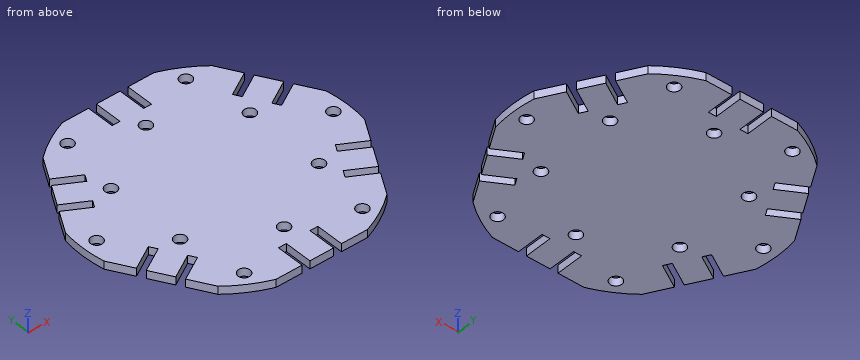
from build123d import *

# Parameters (mm, degrees)
MODEL_R             = 1.5
BOSS_EXTRUDE1_DEPTH = 2


with BuildPart() as part:
    # Model → Boss-Extrude1 (new body)
    with BuildSketch(Plane.XY):
        with BuildLine():
            Line((-18.701410202, -16.570766906), (-19.701410202, -14.838716098))
            Line((-19.701410202, -14.838716098), (-25.711054778, -18.308386013))
            Line((-25.711054778, -18.308386013), (-28.711054778, -13.11223359))
            Line((-28.711054778, -13.11223359), (-22.701410202, -9.642563676))
            Line((-22.701410202, -9.642563676), (-23.701410202, -7.910512868))
            Line((-23.701410202, -7.910512868), (-29.711054778, -11.380182782))
            Line((-29.711054778, -11.380182782), (-33.02041498, -5.648202773))
            ThreePointArc((-33.02041498, -5.648202773), (-33.5, 0), (-33.02041498, 5.648202773))
            Line((-33.02041498, 5.648202773), (-29.711054778, 11.380182782))
            Line((-29.711054778, 11.380182782), (-23.701410202, 7.910512868))
            Line((-23.701410202, 7.910512868), (-22.701410202, 9.642563676))
            Line((-22.701410202, 9.642563676), (-28.711054778, 13.11223359))
            Line((-28.711054778, 13.11223359), (-25.711054778, 18.308386013))
            Line((-25.711054778, 18.308386013), (-19.701410202, 14.838716098))
            Line((-19.701410202, 14.838716098), (-18.701410202, 16.570766906))
            Line((-18.701410202, 16.570766906), (-24.711054778, 20.04043682))
            Line((-24.711054778, 20.04043682), (-21.401694577, 25.77241683))
            ThreePointArc((-21.401694577, 25.77241683), (-16.75, 29.011851027), (-11.618720403, 31.420619602))
            Line((-11.618720403, 31.420619602), (-5, 31.420619602))
            Line((-5, 31.420619602), (-5, 24.481279774))
            Line((-5, 24.481279774), (-3, 24.481279774))
            Line((-3, 24.481279774), (-3, 31.420619602))
            Line((-3, 31.420619602), (3, 31.420619602))
            Line((3, 31.420619602), (3, 24.481279774))
            Line((3, 24.481279774), (5, 24.481279774))
            Line((5, 24.481279774), (5, 31.420619602))
            Line((5, 31.420619602), (11.618720403, 31.420619602))
            ThreePointArc((11.618720403, 31.420619602), (16.75, 29.011851027), (21.401694577, 25.77241683))
            Line((21.401694577, 25.77241683), (24.711054778, 20.04043682))
            Line((24.711054778, 20.04043682), (18.701410202, 16.570766906))
            Line((18.701410202, 16.570766906), (19.701410202, 14.838716098))
            Line((19.701410202, 14.838716098), (25.711054778, 18.308386013))
            Line((25.711054778, 18.308386013), (28.711054778, 13.11223359))
            Line((28.711054778, 13.11223359), (22.701410202, 9.642563676))
            Line((22.701410202, 9.642563676), (23.701410202, 7.910512868))
            Line((23.701410202, 7.910512868), (29.711054778, 11.380182782))
            Line((29.711054778, 11.380182782), (33.02041498, 5.648202773))
            ThreePointArc((33.02041498, 5.648202773), (33.5, 0), (33.02041498, -5.648202773))
            Line((33.02041498, -5.648202773), (29.711054778, -11.380182782))
            Line((29.711054778, -11.380182782), (23.701410202, -7.910512868))
            Line((23.701410202, -7.910512868), (22.701410202, -9.642563676))
            Line((22.701410202, -9.642563676), (28.711054778, -13.11223359))
            Line((28.711054778, -13.11223359), (25.711054778, -18.308386013))
            Line((25.711054778, -18.308386013), (19.701410202, -14.838716098))
            Line((19.701410202, -14.838716098), (18.701410202, -16.570766906))
            Line((18.701410202, -16.570766906), (24.711054778, -20.04043682))
            Line((24.711054778, -20.04043682), (21.401694577, -25.77241683))
            ThreePointArc((21.401694577, -25.77241683), (16.75, -29.011851027), (11.618720403, -31.420619602))
            Line((11.618720403, -31.420619602), (5, -31.420619602))
            Line((5, -31.420619602), (5, -24.481279774))
            Line((5, -24.481279774), (3, -24.481279774))
            Line((3, -24.481279774), (3, -31.420619602))
            Line((3, -31.420619602), (-3, -31.420619602))
            Line((-3, -31.420619602), (-3, -24.481279774))
            Line((-3, -24.481279774), (-5, -24.481279774))
            Line((-5, -24.481279774), (-5, -31.420619602))
            Line((-5, -31.420619602), (-11.618720403, -31.420619602))
            ThreePointArc((-11.618720403, -31.420619602), (-16.75, -29.011851027), (-21.401694577, -25.77241683))
            Line((-21.401694577, -25.77241683), (-24.711054778, -20.04043682))
            Line((-24.711054778, -20.04043682), (-18.701410202, -16.570766906))
        make_face()
        with Locations((-17.610482102, -10.167416582)):
            Circle(MODEL_R, mode=Mode.SUBTRACT)
        with Locations((-17.610482102, 10.167416582)):
            Circle(MODEL_R, mode=Mode.SUBTRACT)
        with Locations((0, -20.334833165)):
            Circle(MODEL_R, mode=Mode.SUBTRACT)
        with Locations((17.610482102, -10.167416582)):
            Circle(MODEL_R, mode=Mode.SUBTRACT)
        with Locations((0, 20.334833165)):
            Circle(MODEL_R, mode=Mode.SUBTRACT)
        with Locations((-30, 0)):
            Circle(MODEL_R, mode=Mode.SUBTRACT)
        with Locations((-15, -25.980762114)):
            Circle(MODEL_R, mode=Mode.SUBTRACT)
        with Locations((15, 25.980762114)):
            Circle(MODEL_R, mode=Mode.SUBTRACT)
        with Locations((-15, 25.980762114)):
            Circle(MODEL_R, mode=Mode.SUBTRACT)
        with Locations((15, -25.980762114)):
            Circle(MODEL_R, mode=Mode.SUBTRACT)
        with Locations((30, 0)):
            Circle(MODEL_R, mode=Mode.SUBTRACT)
        with Locations((17.610482102, 10.167416582)):
            Circle(MODEL_R, mode=Mode.SUBTRACT)
    extrude(amount=BOSS_EXTRUDE1_DEPTH)


solid = part.part
Verification items for the finished model (mm, model axes). Give positions to 0.01 mm unless a question says otherwise; leave off trailing zeros. Loops run counter-clockwise (first coordinate to the right, second up) from the corner with the lowest first, then second, coordinate; pieces in that order, holes last. Notation, with made-up numbers: (16, 59) - (55, 59) arc R21 ccw to (55, 75) - close; hole circle Ø9 at (30.5, -34). An arc over 180 degrees is marked (long way). Write each question's results on one line, items separated by ' | '.
1) Sectioned sample at C-C on z = 1.35. Count the separate pieces of the cut face and the enclosed holes in it, plus the area to 3 significant figures.
Solution:
separate pieces: 1 | enclosed holes: 12 | area: 3,080 mm2
2) Material ranges on L1, parallel to Y at x = 0, z = 1.65; L2, parallel to X at y = -26, z = 1.95; L3, parallel to Y at x = -22.5, z = 0.8, recorded low to high. Write a range as from..to.
Solution:
L1: -31.42..-21.83, -18.83..18.83, 21.83..31.42 | L2: -21.12..-16.5, -13.5..-5, -3..3, 5..13.5, 16.5..21.12 | L3: -23.87..-18.76, -16.45..16.45, 18.76..23.87
3) Sectioned sample at B-B on y = 0. Record the boundary of the cut face in (x, z).
Solution:
outline: (-33.5, 0) - (-31.5, 0) - (-31.5, 2) - (-33.5, 2) - close; (-28.5, 0) - (28.5, 0) - (28.5, 2) - (-28.5, 2) - close; (31.5, 0) - (33.5, 0) - (33.5, 2) - (31.5, 2) - close
4) Sectioned sample at A-A on x = 0. Record the boundary of the cut face in (y, z).
Solution:
outline: (-31.42, 0) - (-21.83, 0) - (-21.83, 2) - (-31.42, 2) - close; (-18.83, 0) - (18.83, 0) - (18.83, 2) - (-18.83, 2) - close; (21.83, 0) - (31.42, 0) - (31.42, 2) - (21.83, 2) - close
5) Depth check by flat-ended pin: P1, Ø0.6, axis at y = 29.5, z = 1.5, coming from the +X side; P2, Ø0.6, axis at y = -27, z = 1, coming from the -X side; P3, Ø1, axis at x = 12.5, z = 1, coming from the -Y side; P4, Ø8, axis at x = 4, y = 16.5, coming from the -Z side. Enter the tip coordinate at first touch or a pass-through.
Solution:
P1: x = 16.42 | P2: x = -20.23 | P3: y = -31.28 | P4: z = 0
